For this review, take the finished solid that the model builds, in its own axes (mm). A direction names the side the tool comes from. Coordinates: 2 decimals unless noted, no trailing zeros. Order: outer loops, then holes, each group sorted by start corner. A loop starts at its lowest first (then second) coordinate and runs counter-clockwise, first axis right, second up. Notation, with made-up numbers: (-18, 75) -> (38, 75) arc R31 cw to (38, 103) -> close; hole circle Ø2 at (7, -23). An arc over 180 degrees is marked (long way). Return JSON: item names as keys, results as strings. Group by question number.
Item 1: Take a section at B-B (z = 14.5). Write out the cut boundary in (x, y), then the cut area to 3 significant figures.
Item 2: Draft analysis for pull direction Y (two halves, no side actions). For faces 3 (the cylindrical face through (12.5, -4.9, 1)), 4 (the flat face through (29, -10, 1)), 5 (the flat face through (43, -4.9, 11.5)), state which applies: +Y half, -Y half, draft (parallel to the pull), parting line (faces both ways), or undercut.
Item 3: Take a section at A-A (y = -5). Write out the cut boundary in (x, z).
Item 4: For line 1 along Y through (x, z) = (43.5, 14.5); line 2 along Z through (x, y) = (10, -1.5); line 3 along X through (y, z) = (-4, 17), list the stretches that pass through material, from the lowest coordinate up.
Item 5: Machinability: for faces 1 (the flat face through (22, -5, 0)), 2 (the flat face through (21, -5, 2)), which of the approach directions +Z, -Z, +X, -X, +Y, -Y give a long, thin tool a straight path to every point of the face, cutting with its end or side? Answer none if there is none.
Item 6: Take a section at D-D (y = -1.5). Write out the cut boundary in (x, z), then the cut area to 3 significant figures.
Item 7: Take a section at C-C (x = 15). Write out the cut boundary in (y, z), then the cut area to 3 significant figures.
Item 8: Insertion check: pin 1 (6 mm diameter, centred on x = 26.5, y = -4, fed in from +Z); pin 2 (2 mm diameter, centred on y = -4, z = 20, fed in from -X); pin 3 (8 mm diameter, centred on x = 22.5, z = 8.5, fed in from +Y). Each pin has a flat end and moves straight along its axis. Give the tip position at first contact, or say it passes through.
Autodesk Inventor part; units mm, degrees
ref_plane "YZ Plane" through (0, 0, 0) normal (1, 0, 0) x (0, 1, 0)
ref_plane "XZ Plane" through (0, 0, 0) normal (0, 1, 0) x (-1, 0, 0)
ref_plane "XY Plane" through (0, 0, 0) normal (0, 0, 1) x (1, 0, 0)
sketch "Sketch1" plane through (0, 0, 0) normal (0, 0, 1) x (1, 0, 0)
  line L0 (0, 0) -> (45, 0)
  line L1 (45, 0) -> (45, -10)
  line L2 (45, -10) -> (0, -10)
  line L3 (0, -10) -> (0, 0)
  line L4 (45, 0) -> (48.2934, 0)
  line L5 (48.2934, 0) -> (48.2934, -10)
  line L6 (48.2934, -10) -> (45, -10)
  line L7 (45, -10) -> (45, 0)
extrude "Extrusion1" add sketch "Sketch1" along normal blind 2 contours L0 L1 L2 L3
sketch "Sketch2" plane through (0, 0, 2) normal (0, 0, 1) x (1, 0, 0)
  line L0 (0, 0) -> (0, -5)
  circle A0 centre (15, -5) radius 2.5
extrude "Extrusion2" cut sketch "Sketch2" against normal blind 2
sketch "Sketch3" plane through (0, 0, 2) normal (0, 0, 1) x (1, 0, 0)
  line L0 (45, -10) -> (45, 0)
  line L1 (45, 0) -> (43, 0)
  line L2 (45, 0) -> (0, 0)
  line L3 (43, 0) -> (43, -10)
  line L4 (0, -10) -> (45, -10)
  line L5 (43, -10) -> (45, -10)
  line L6 (45, -10) -> (45, 0)
  dimension "d10" = 2
extrude "Extrusion3" add sketch "Sketch3" along normal blind 25
sketch "Sketch4" plane through (43, -10, 2) normal (-1, 0, 0) x (0, 0, 1)
  line L0 (25, 0) -> (25, 10)
  circle A0 centre (12.5, 5) radius 2.5
  point P0 (-2, 10)
extrude "Extrusion4" cut sketch "Sketch4" against normal blind 25
properties part number "slider_link" material "Stainless Steel AISI 440C, Welded"
Findings below:
{
 "1": {"outline": "(43, -10) -> (45, -10) -> (45, -7.5) -> (43, -7.5) -> close; (43, -2.5) -> (45, -2.5) -> (45, 0) -> (43, 0) -> close", "area": "10.0 mm2"},
 "2": {"face 3": "undercut", "face 4": "-Y half", "face 5": "draft"},
 "3": {"outline": "(0, 0) -> (12.5, 0) -> (12.5, 2) -> (0, 2) -> close; (17.5, 0) -> (45, 0) -> (45, 12) -> (43, 12) -> (43, 2) -> (17.5, 2) -> close; (43, 17) -> (45, 17) -> (45, 27) -> (43, 27) -> close"},
 "4": {"line 1": "y = -10 to -7.5, -2.5 to 0", "line 2": "z = 0 to 2", "line 3": "x = 43 to 45"},
 "5": {"face 1": "-Z, +X, -X, +Y, -Y", "face 2": "+Z, -X, +Y, -Y"},
 "6": {"outline": "(0, 0) -> (45, 0) -> (45, 27) -> (43, 27) -> (43, 2) -> (0, 2) -> close", "area": "140 mm2"},
 "7": {"outline": "(-10, 0) -> (-7.5, 0) -> (-7.5, 2) -> (-10, 2) -> close; (-2.5, 0) -> (0, 0) -> (0, 2) -> (-2.5, 2) -> close", "area": "10.0 mm2"},
 "8": {"pin 1": "stops at z = 2", "pin 2": "stops at x = 43", "pin 3": "passes through"}
}
